```python
from build123d import *

# Parameters (mm, degrees)
SKETCH1_W               = 25.4
SKETCH1_H               = 25.4
SKETCH1_W_2             = 22.225
SKETCH1_H_2             = 22.225
BOSS_EXTRUDE1_DEPTH     = 63.99895
SKETCH3_R               = 11.1125
CUT_EXTRUDE2_DEPTH      = 71.016538054
CUT_EXTRUDE3_DEPTH      = 71.016538054
CUT_EXTRUDE3_DEPTH_BACK = 71.016538054
SKETCH6_R               = 1.4732
CUT_EXTRUDE4_DEPTH      = 71.016538054
CUT_EXTRUDE4_DEPTH_BACK = 71.016538054
SKETCH7_R               = 1.4732


with BuildPart() as part:
    # Sketch1 → Boss-Extrude1 (new body)
    with BuildSketch(Plane(origin=(0, 0, 0), x_dir=(1, 0, 0), z_dir=(0, 1, 0))):
        Rectangle(SKETCH1_W, SKETCH1_H)
        Rectangle(SKETCH1_W_2, SKETCH1_H_2, mode=Mode.SUBTRACT)
    extrude(amount=BOSS_EXTRUDE1_DEPTH)

    # Sketch3 → Cut-Extrude2 (cut, through all)
    with BuildSketch(Plane(origin=(12.7, 0, 0), x_dir=(0, 0, -1), z_dir=(1, 0, 0))):
        with Locations((0, 33.3375)):
            Circle(SKETCH3_R)
    extrude(amount=-CUT_EXTRUDE2_DEPTH, mode=Mode.SUBTRACT)

    # Sketch6 → Cut-Extrude3 (cut, two sides: drawn at the far end of the back side and taken through both)
    with BuildSketch(Plane(origin=(0, 0, -12.7), x_dir=(-1, 0, 0), z_dir=(0, 0, -1)).offset(-CUT_EXTRUDE3_DEPTH_BACK)):
        with Locations((8.889941847, 55.381049815)):
            Circle(SKETCH6_R)
    extrude(amount=CUT_EXTRUDE3_DEPTH + CUT_EXTRUDE3_DEPTH_BACK, mode=Mode.SUBTRACT)

    # Sketch7 → Cut-Extrude4 (cut, two sides: drawn at the far end of the back side and taken through both)
    with BuildSketch(Plane(origin=(0, 0, -12.7), x_dir=(-1, 0, 0), z_dir=(0, 0, -1)).offset(-CUT_EXTRUDE4_DEPTH_BACK)):
        with Locations((-8.889941847, 55.381049816)):
            Circle(SKETCH7_R)
    extrude(amount=CUT_EXTRUDE4_DEPTH + CUT_EXTRUDE4_DEPTH_BACK, mode=Mode.SUBTRACT)


solid = part.part
```
Check sheet for the modelled part. Datum: model origin and axes. Units: mm. A direction names the side the tool comes from. Round coordinates to 2 decimals unless told otherwise and drop trailing zeros. Loops run counter-clockwise (first coordinate to the right, second up) from the corner with the lowest first, then second, coordinate; pieces in that order, holes last. Notation, with made-up numbers: (-25.75, 74) - (7.25, 74) arc R13 ccw to (7.25, 92) - close; hole circle Ø2 at (63, -35). An arc over 180 degrees is marked (long way). Write item = value, one per line. Start each with the question number.
Q1. Depth check by flat-ended pin: P1, Ø2.5, axis at x = -8.89, y = 55.38, coming from the +Z side. Enter the tip coordinate at first touch or a pass-through.
Q2. Release check for a two-part mould opening along X. For faces 1 (the face through (-12.7, 24, -8)), 2 (the face through (-10.25, 54.82, 11.92)), 3 (the face through (0, 32, 12.7)), 4 (the face through (12.7, 24, -8)) record: pulls with the +X half, pulls with the -X half, needs draft (parallel to the pull), parting line crosses it, or undercut.
Q3. Section check D-D (x = 9). Record the boundary of the cut face in (y, z).
Q4. Section check A-A (z = 0). Count the separate pieces of the cut face and the enclosed holes in it, plus the area to 3 significant figures.
Q5. Thickness scan on L1, parallel to Z at x = 0, y = 31; L2, parallel to Y at x = -12.25, z = 0 (3 decimals). Record the ranges inside material, lowest first.
Q6. Section check B-B (x = 4). Record the boundary of the cut face in (y, z).
Q7. Section check C-C (y = 12). Record the boundary of the cut face in (x, z), plus the area to 3 significant figures.
Q8. Access from +Z, -Z, +X, -X, +Y, -Y to the whole of each face (thin tool, end or side, straight path). Record for faces 5 (the face through (0, 32, -12.7)), 6 (the face through (0, 32, -11.112)).
Derived:
q1.P1 = through
q2.face_1 = pulls with the -X half
q2.face_2 = undercut
q2.face_3 = needs draft
q2.face_4 = pulls with the +X half
q3.outline = (0, -12.7) - (53.91, -12.7) - (53.91, -11.11) - (0, -11.11) - close; (0, 11.11) - (53.91, 11.11) - (53.91, 12.7) - (0, 12.7) - close; (56.85, -12.7) - (64, -12.7) - (64, -11.11) - (56.85, -11.11) - close; (56.85, 11.11) - (64, 11.11) - (64, 12.7) - (56.85, 12.7) - close
q4.separate_pieces = 4
q4.enclosed_holes = 0
q4.area = 133 mm^2
q5.L1 = -12.7 to -11.11, 11.11 to 12.7
q5.L2 = 0 to 22.225, 44.45 to 63.999
q6.outline = (0, -12.7) - (64, -12.7) - (64, -11.11) - (0, -11.11) - close; (0, 11.11) - (64, 11.11) - (64, 12.7) - (0, 12.7) - close
q7.outline = (-12.7, -12.7) - (12.7, -12.7) - (12.7, 12.7) - (-12.7, 12.7) - close; hole (-11.11, -11.11) - (11.11, -11.11) - (11.11, 11.11) - (-11.11, 11.11) - close
q7.area = 151 mm^2
q8.face_5 = -Z, +X, -X, +Y, -Y
q8.face_6 = +Y, -Y
